Drawing for the job (mm, zero at the part's lowest x, y, z). A direction names the side the tool comes from. Round coordinates to 2 decimals unless told otherwise and drop trailing zeros. Loops run counter-clockwise (first coordinate to the right, second up) from the corner with the lowest first, then second, coordinate; pieces in that order, holes last. Notation, with made-up numbers: M -25,80 L 16,80 A36 ccw 16,116 Z; hole C 38,87.25 d6. An arc over 180 degrees is marked long. Answer in a Markdown table with one row per item.
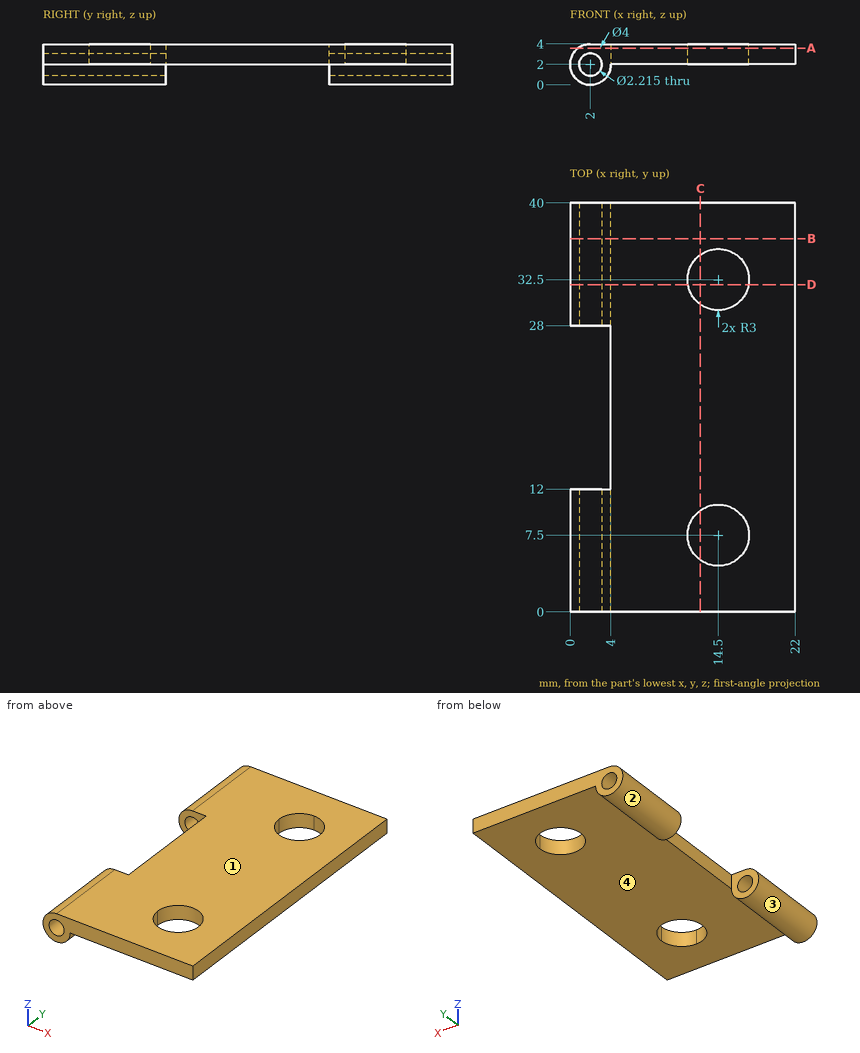
1. Saw through at C-C (x = 12.75). Write the cut outline in (y, z).
Verdict:
| item | result |
|---|---|
| outline | M 0,2 L 5.06,2 L 5.06,4 L 0,4 Z; M 9.94,2 L 30.06,2 L 30.06,4 L 9.94,4 Z; M 34.94,2 L 40,2 L 40,4 L 34.94,4 Z |
2. Tool access for the marked faces 3 and 4: list every direction of +Z, -Z, +X, -X, +Y, -Y with a clear straight run to the whole face (end or side of a thin tool).
Verdict:
| item | result |
|---|---|
| face 3 | +Y, -Y |
| face 4 | -Z, +X, +Y, -Y |
3. Wall check: probe 1 along Z at (x, y) = (2, 6); probe 2 along Y at (x, z) = (16, 3.6); probe 3 along Z at (x, y) = (12.5, 29.5). Give the ranges that are in metal, low to high.
Verdict:
| item | result |
|---|---|
| probe 1 | z = 0 to 0.89, 3.11 to 4 |
| probe 2 | y = 0 to 4.9, 10.1 to 29.9, 35.1 to 40 |
| probe 3 | z = 2 to 4 |
4. Mould opens along X. For the marked faces 1 and 2 say: +X half, -X half, draft (parallel to the pull), parting line (faces both ways), or undercut.
Verdict:
| item | result |
|---|---|
| face 1 | draft |
| face 2 | parting line |
5. Saw through at A-A (z = 3.6). Write the cut outline in (x, y), and give its area (3 significant figures).
Verdict:
| item | result |
|---|---|
| outline | M 0.8,0 L 22,0 L 22,40 L 0.8,40 L 0.8,28 L 4,28 L 4,12 L 0.8,12 Z; hole C 14.5,7.5 d6; hole C 14.5,32.5 d6 |
| area | 740 mm² |
6. Saw through at B-B (y = 36.5). Write the cut outline in (x, z) (1 decimal).
Verdict:
| item | result |
|---|---|
| outline | M 2,4 A2 ccw long 4,2 L 22,2 L 22,4 Z; hole C 2,2 d2.2 |
7. Saw through at D-D (y = 32). Write the cut outline in (x, z) (1 decimal).
Verdict:
| item | result |
|---|---|
| outline | M 2,4 A2 ccw long 4,2 L 11.5,2 L 11.5,4 Z; M 17.5,2 L 22,2 L 22,4 L 17.5,4 Z; hole C 2,2 d2.2 |
8. Pin check, flat tips, straight feed: pin 1 (9 mm diameter, centred on x = 10, y = 26, fed in from -Z); pin 2 (1 mm diameter, centred on x = 5.5, z = 1, fed in from +Y); pin 3 (1.2 mm diameter, centred on x = 3, z = 1, fed in from -Y); pin 4 (1 mm diameter, centred on y = 19.5, z = 3.5, fed in from -X). Stop position of each tip, or through.
Verdict:
| item | result |
|---|---|
| pin 1 | stops at z = 2 |
| pin 2 | passes through |
| pin 3 | stops at y = 0 |
| pin 4 | stops at x = 4 |
